Check sheet for the modelled part. Datum: model origin and axes. Units: mm. Round coordinates to 2 decimals unless told otherwise and drop trailing zeros. Write each loop counter-clockwise with the first axis right and the second up, starting at its lowest first coordinate (ties: lowest second). Pieces come first, ordered by that corner, then holes.
Item 1: Material ranges on line 1 along Z through (x, y) = (-10.5, 0.4); line 2 along X through (y, z) = (0.05, 43), recorded low to high.
Item 2: Section check A-A, the plane y = 0.35. Record the cut outline in (x, z).
Item 3: Depth check by flat-ended pin: pin 1 (0.5 mm diameter, centred on x = -8, y = 0.5, fed in from +Z); pin 2 (0.5 mm diameter, centred on y = 0.5, z = 15, fed in from -X). Enter the tip coordinate at first touch or a pass-through.
Item 4: Section check C-C, the plane z = 44.5. Record the cut outline in (x, y), plus the area to 3 significant figures.
Item 5: Section check B-B, the plane x = -10. Record the cut outline in (y, z).
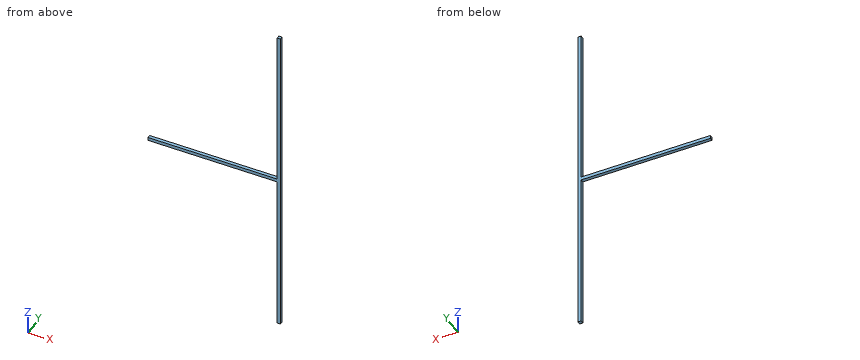
Autodesk Fusion 360 part; units mm, degrees
sketch "Sketch1" plane through (0, 0, 0) normal (0, 1, 0) x (1, 0, 0)
  line L0 (0, 0) -> (17, 0)
  line L1 (17, 0) -> (17, -1)
  line L2 (17, -1) -> (0, -1)
  line L3 (0, -1) -> (0, 0)
  line L4 (17, -1) -> (17, -0.5)
  line L5 (17, -0.5) -> (17.5, -0.5)
  line L6 (18, 24.5) -> (17, 24.5)
  line L7 (17, 24.5) -> (17, -25.5)
  line L8 (17, -25.5) -> (18, -25.5)
  line L9 (18, -25.5) -> (18, 24.5)
  point P0 (17.5, -0.5)
  dimension "d1" = 17
  dimension "d2" = 1
  dimension "d3" = 1
  dimension "d4" = 50
extrude "Extrude1" add sketch "Sketch1" along normal blind 1
extrude "Extrude2" add 1 faces at (0, 0.3333, 0.6667) along direction (-1, 0, 0) blind 5
extrude "Extrude3" add 1 faces at (-5, 0.3333, 0.6667) along direction (-1, 0, 0) blind 18
extrude "Extrude4" add 1 faces at (17.3333, 0.3333, 25.5) along direction (0, 0, 1) blind 25
extrude "Extrude5" add 1 faces at (17.6667, 0.3333, -24.5) along direction (0, 0, -1) blind 25
Values found:
1. line 1: z = 0 to 1
1. line 2: x = 17 to 18
2. outline: (-23, 0) - (17, 0) - (17, -49.5) - (18, -49.5) - (18, 50.5) - (17, 50.5) - (17, 1) - (-23, 1) - close
3. pin 1: stops at z = 1
3. pin 2: stops at x = 17
4. outline: (17, 0) - (18, 0) - (18, 1) - (17, 1) - close
4. area: 1.00 mm2
5. outline: (0, 0) - (1, 0) - (1, 1) - (0, 1) - close
